Geometry: final body of the model. Coordinates: model frame, mm. A direction names the side the tool comes from. Coordinates: 2 decimals unless noted, no trailing zeros. Loops run counter-clockwise (first coordinate to the right, second up) from the corner with the lowest first, then second, coordinate; pieces in that order, holes last. Notation, with made-up numbers: (32, -35.5) -> (52, -35.5) arc R10 ccw to (52, -25.5) -> close; hole circle Ø5 at (86, 63.25). An arc over 180 degrees is marked (long way). One line per item, written item: value. Start each with the question number.
Item 1: Section query A-A on z = -5. Return loops of the section in (x, y).
Item 2: Ray query, probe 1 along Y at (x, z) = (0, -0.65); probe 2 along Y at (x, z) = (2.5, -11); probe 3 along Z at (x, y) = (8, 10.5). Return the intervals inside material, ascending. Write a range as from..to.
Item 3: Section query B-B on x = 0. Return loops of the section in (y, z), then the cut area to 3 significant figures.
Item 4: Section query C-C on y = 7. Return loops of the section in (x, z), then the cut area to 3 significant figures.
Item 5: Mould query, pull axis Z, two halves, no side actions, for faces 3 (the flat face through (-10, 0.4, -5.6)), 4 (the flat face through (0, 11, -1)), 5 (the cylindrical face through (0.088, 0.493, -3.002)). Classes: +Z half, -Z half, draft (parallel to the pull), parting line (faces both ways), or undercut.
Item 6: Set-up query: faces 1 (the cylindrical face through (-0.26, 16.983, -0.493)), 2 (the flat face through (0, 1, -10)). Return all of +Z, -Z, +X, -X, +Y, -Y with unobstructed straight access to the full face (end or side cutting, diameter ignored); none if empty.
Item 7: Contact query for flat-ended pins moving along their axis: pin 1 Ø5 at (x, y) = (0, 15) entering from -Z; pin 2 Ø10 at (x, y) = (-6.5, 15) entering from +Z; pin 3 Ø1 at (x, z) = (-4, -14) entering from +Y. Output: stop coordinate, or through.
Item 8: Section query D-D on x = 8. Return loops of the section in (y, z).
from build123d import *

# Parameters (mm, degrees)
BOSS_EXTRUDE1_DEPTH = 10
SKETCH2_R           = 2
CUT_EXTRUDE1_DEPTH  = 20
SKETCH3_R           = 2
CUT_EXTRUDE2_DEPTH  = 20


with BuildPart() as part:
    # Sketch1 → Boss-Extrude1 (new, symmetric)
    with BuildSketch(Plane(origin=(0, 0, 0), x_dir=(0, 0, -1), z_dir=(1, 0, 0))):
        with BuildLine():
            Line((20, 0), (1, 0))
            ThreePointArc((1, 0), (0.292893219, 0.292893219), (0, 1))
            Line((0, 1), (0, 20))
            Line((0, 20), (1, 20))
            Line((1, 20), (1, 1))
            Line((1, 1), (20, 1))
            Line((20, 1), (20, 0))
        make_face()
    extrude(amount=BOSS_EXTRUDE1_DEPTH, both=True)

    # Sketch2 → Cut-Extrude1 (cut)
    with BuildSketch(Plane.XY):
        with Locations((0, 7)):
            Circle(SKETCH2_R)
        with Locations((0, 15)):
            Circle(SKETCH2_R)
    extrude(amount=-CUT_EXTRUDE1_DEPTH, mode=Mode.SUBTRACT)

    # Sketch3 → Cut-Extrude2 (cut)
    with BuildSketch(Plane.XZ):
        with Locations(Location((0, -13, 0), (0, 0, 270))):
            Circle(SKETCH3_R)
        with Locations(Location((0, -5, 0), (0, 0, 270))):
            Circle(SKETCH3_R)
    extrude(amount=-CUT_EXTRUDE2_DEPTH, mode=Mode.SUBTRACT)


solid = part.part
Reply:
1. outline: (-10, 0) -> (-2, 0) -> (-2, 1) -> (-10, 1) -> close; (2, 0) -> (10, 0) -> (10, 1) -> (2, 1) -> close
2. probe 1: y = 0.06..5, 9..13, 17..20
2. probe 2: y = 0..1
2. probe 3: z = -1..0
3. outline: (0, -20) -> (1, -20) -> (1, -15) -> (0, -15) -> close; (0, -11) -> (1, -11) -> (1, -7) -> (0, -7) -> close; (0, -3) -> (1, -3) -> (1, -1) -> (5, -1) -> (5, 0) -> (1, 0) arc R1 ccw to (0, -1) -> close; (9, -1) -> (13, -1) -> (13, 0) -> (9, 0) -> close; (17, -1) -> (20, -1) -> (20, 0) -> (17, 0) -> close
3. area: 22.8 mm²
4. outline: (-10, -1) -> (-2, -1) -> (-2, 0) -> (-10, 0) -> close; (2, -1) -> (10, -1) -> (10, 0) -> (2, 0) -> close
4. area: 16.0 mm²
5. face 3: draft
5. face 4: -Z half
5. face 5: undercut
6. face 1: +Z, -Z
6. face 2: -Z, +X, -X, +Y
7. pin 1: stops at z = -1
7. pin 2: stops at z = 0
7. pin 3: stops at y = 1
8. outline: (0, -20) -> (1, -20) -> (1, -1) -> (20, -1) -> (20, 0) -> (1, 0) arc R1 ccw to (0, -1) -> close
